Could you check a few things on this model? Use its own coordinates, in mm. A direction names the side the tool comes from. Coordinates: 2 decimals unless noted, no trailing zeros. Loops run counter-clockwise (first coordinate to the right, second up) from the corner with the lowest first, then second, coordinate; pieces in that order, holes last. Notation, with made-up numbers: (79.5, 80) - (130.5, 80) arc R15 cw to (130.5, 96) - close; hole circle Ø7 at (55.25, 38.5). An arc over 180 degrees is marked (long way). One line per question, with ' | ' between items. Start each with the question number.
1. Which directions (+Z, -Z, +X, -X, +Y, -Y) give clear straight access to the entire face, cutting with the end or side of a thin tool? Please do faces 5 (the flat face through (63.202, 0, 37)), 6 (the flat face through (-1, 30, 40)).
2. I want a section at A-A, the plane x = 19. Write out the boundary of the cut face in (y, z).
3. I want a section at B-B, the plane z = 60. Write out the boundary of the cut face in (x, y), then the cut area to 3 significant figures.
4. I'm going to push a flat-ended pin straight in: P1, Ø18, axis at x = 13.5, y = 0, coming from the +Z side. Where does the tip first touch, or does it pass through?
5. We'd pull the mould along X, two halves only. Please class faces 1 (the flat face through (-57.5, 0, 40)), 2 (the flat face through (-63.202, 0, 37)), 3 (the flat face through (-1, -35.56, 37)), 4 (the flat face through (57.5, 0, 40)): pulls with the +X half, pulls with the -X half, needs draft (parallel to the pull), parting line crosses it, or undercut.
6. Please list where these lines run through material, in increasing order: L1, parallel to X at y = 8, z = 19.5; L2, parallel to X at y = -32.1, z = 37.5; L3, parallel to Z at x = 0, y = -33.35. Write a range as [from, to].
7. I want a section at C-C, the plane y = 9.5. Write out the boundary of the cut face in (x, z).
from build123d import *

# Parameters (mm, degrees)
F0_W     = 115
F0_H     = 60
F2_DEPTH = 5
F1_W     = 126.404688
F1_H     = 71.120002
F1_W_2   = 115
F1_H_2   = 60
F3_DEPTH = 75
F4_R     = 0.08
F5_DEPTH = 7.5438


with BuildPart() as f2:
    # F0 (on Top) → F2 (new body)
    with BuildSketch(Plane.XY):
        Rectangle(F0_W, F0_H)
    extrude(amount=F2_DEPTH)

    # F1 (on face) → F3 (join)
    with BuildSketch(Plane.XY):
        Rectangle(F1_W, F1_H)
        Rectangle(F1_W_2, F1_H_2, mode=Mode.SUBTRACT)
    extrude(amount=F3_DEPTH)

    # F4 (on face) → F5 (cut)
    with BuildSketch(Plane.XZ.offset(35.560001)):
        with Locations((0, 37.5)):
            Circle(F4_R)
    extrude(amount=-F5_DEPTH, mode=Mode.SUBTRACT)


solid = f2.part
Results are:
1) face 5: +Z, -Z, +X, +Y, -Y | face 6: +Z
2) outline: (-35.56, 0) - (35.56, 0) - (35.56, 75) - (30, 75) - (30, 5) - (-30, 5) - (-30, 75) - (-35.56, 75) - close
3) outline: (-63.2, -35.56) - (63.2, -35.56) - (63.2, 35.56) - (-63.2, 35.56) - close; hole (-57.5, -30) - (57.5, -30) - (57.5, 30) - (-57.5, 30) - close | area: 2,090 mm2
4) P1: stops at z = 5
5) face 1: undercut | face 2: pulls with the -X half | face 3: needs draft | face 4: undercut
6) L1: x = [-63.2, -57.5], [57.5, 63.2] | L2: x = [-63.2, -0.08], [0.08, 63.2] | L3: z = [0, 37.42], [37.58, 75]
7) outline: (-63.2, 0) - (63.2, 0) - (63.2, 75) - (57.5, 75) - (57.5, 5) - (-57.5, 5) - (-57.5, 75) - (-63.2, 75) - close
